Source: CAD feature listing. Evaluate the final solid. Frame: model axes, mm. Face numbers are marked on the shaded views. A direction names the side the tool comes from. Give positions to 0.01 mm unless a question says otherwise; leave off trailing zeros. Order: outer loops, then holes, each group sorted by start corner. A loop starts at its lowest first (then second) coordinate and runs counter-clockwise, first axis right, second up.
Autodesk Inventor part; units mm, degrees
ref_plane "Work Plane1" through (45, -30, 10) normal (0.7071, 0, -0.7071) x (0, 1, 0)
ref_plane "Work Plane2" through (0, 30, 0) normal (0, 1, 0) x (-1, 0, 0)
ref_plane "Work Plane3" through (0, -30, 0) normal (0, 1, 0) x (-1, 0, 0)
sketch "Sketch1" plane through (0, 0, 0) normal (0, 0, 1) x (1, 0, 0)
  line L0 (-363.8821, 101.7163) -> (-138.7473, 103.6763) construction
  line L1 (-138.7473, 103.6763) -> (-137.081, -87.7242) construction
  line L2 (-137.081, -87.7242) -> (-362.2158, -89.6841) construction
  line L3 (-362.2158, -89.6841) -> (-363.8821, 101.7163) construction
  line L4 (-45, 30) -> (45, 30)
  line L5 (45, 30) -> (45, -30)
  line L6 (-45, -30) -> (-45, 30)
  line L7 (-45, 30) -> (45, -30) construction
  line L8 (45, 30) -> (-45, -30) construction
  arc A0 (24, 0) -> (6, 0) centre (15, 0) ccw
  line L9 (15, 0) -> (6, 0) construction
  line L10 (15, 0) -> (24, 0) construction
  line L11 (6, 0) -> (6, -30)
  line L12 (24, 0) -> (24, -30)
  line L13 (45, -30) -> (24, -30)
  line L14 (6, -30) -> (-45, -30)
  point P0 (0, 0)
  dimension "d9" = 90
  dimension "d10" = 60
  dimension "d12" = 9
  dimension "d13" = 180
  dimension "d14" = 30
  dimension "d15" = 30
extrude "Extrusion1" add sketch "Sketch1" along normal blind 10
ref_plane "Work Plane1" through (45, -30, 10) normal (0.7071, 0, -0.7071) x (0, 1, 0)
sketch "Sketch2" plane through (45, -30, 10) normal (0.7071, 0, -0.7071) x (0, 1, 0)
  line L0 (60, 0) -> (60, -63.6396)
  line L1 (0, 0) -> (60, 0)
  circle A0 centre (30, 45.5) radius 7.5
  line L2 (60, 0) -> (36.9322, 55.8626)
  line L3 (0, 0) -> (23.0678, 55.8626)
  arc A1 (36.9322, 55.8626) -> (23.0678, 55.8626) centre (30, 53) ccw
  point P0 (30, -38.8909)
  dimension "d19" = 15
  dimension "d20" = 45.5
  dimension "d22" = 7.5
extrude "Extrusion2" add sketch "Sketch2" along normal blind 10
sketch "Sketch3" plane through (0, 0, 0) normal (0, 1, 0) x (-1, 0, 0)
  point P0 (0, 0)
sketch "Sketch4" plane through (0, 0, 0) normal (0, 0, 1) x (1, 0, 0)
  point P0 (0, 0)
sketch "Sketch5" plane through (0, 0, 0) normal (0, 1, 0) x (-1, 0, 0)
  point P0 (0, 0)
ref_plane "Work Plane2" through (0, 30, 0) normal (0, 1, 0) x (-1, 0, 0)
ref_plane "Work Plane3" through (0, -30, 0) normal (0, 1, 0) x (-1, 0, 0)
sketch "Sketch6" plane through (0, 30, 0) normal (0, 1, 0) x (-1, 0, 0)
  line L0 (-45, 0) -> (-45, 10)
  line L1 (-45, 10) -> (-52.0711, 2.9289)
  line L2 (-45, 0) -> (-52.0711, 2.9289)
  line L3 (-52.0711, 2.9289) -> (-45, 10)
  line L4 (-45, 10) -> (-45, 0)
  point P0 (0, 0)
sketch "Sketch7" plane through (0, -30, 0) normal (0, 1, 0) x (-1, 0, 0)
  point P0 (0, 0)
sketch "Sketch8" plane through (0, -30, 0) normal (0, 1, 0) x (-1, 0, 0)
  line L0 (-45, 10) -> (-52.0711, 2.9289)
  line L1 (-52.0711, 2.9289) -> (-45, 10)
  line L2 (-45, 0) -> (-45, 10)
  line L3 (-45, 10) -> (-45, 0)
  line L4 (-45, 0) -> (-52.0711, 2.9289)
  point P0 (0, 0)
loft "Loft1" add profiles "Sketch8", "Sketch6"
sketch "Sketch9" plane through (0, 0, 10) normal (0, 0, 1) x (1, 0, 0)
  line L0 (45, 30) -> (-45, 30)
  line L1 (-45, 30) -> (-105, 30)
  line L2 (-45, 30) -> (-45, -30)
  line L3 (-45, -30) -> (-105, -30)
  arc A0 (-45, -30) -> (-45, 30) centre (-45, 0) ccw
  arc A1 (-57, -9) -> (-57, 9) centre (-45, 0) ccw
  line L4 (-57, 9) -> (-105, 9)
  line L5 (-57, -9) -> (-105, -9)
  line L6 (-105, -30) -> (-105, -9)
  line L7 (-105, 9) -> (-105, 30)
  point P0 (0, 0)
  dimension "d31" = 60
  dimension "d32" = 60
  dimension "d33" = 15
  dimension "d34" = 18
  dimension "d35" = 21
extrude "Extrusion3" add sketch "Sketch9" along normal blind 17.5 and the other way blind 27.5 contours L2 A1 L4 L7 L1 | A0 L2 A1 | L3 L6 L5 A1 L2
sketch "Sketch10" plane through (-105, 9, 27.5) normal (-1, 0, 0) x (0, 0, 1)
  line L0 (-45, 0) -> (-45, 21)
  line L1 (0, 21) -> (0, 0)
  point P0 (-27.5, -9)
  point P1 (-45, 10.5)
  dimension "d40" = 45
sketch "Sketch11" plane through (-45, 30, 0) normal (0, 1, 0) x (1, 0, 0)
  circle A0 centre (-38.4851, -5) radius 12
  line L0 (0, -27.5) -> (-60, -27.5)
  point P0 (45, 0)
  dimension "d42" = 24
extrude "Extrusion4" cut sketch "Sketch11" against normal blind 9.5
sketch "Sketch12" plane through (-83.4851, 20.5, 5) normal (0, 1, 0) x (1, 0, 0)
  circle A0 centre (0, 0) radius 12
  circle A1 centre (0, 0) radius 6
  point P0 (83.4851, 5)
  dimension "d46" = 12
extrude "Extrusion5" cut sketch "Sketch12" against normal blind 12 contours A1
sketch "Sketch13" plane through (6, -30, 0) normal (0, -1, 0) x (1, 0, 0)
  circle A0 centre (-89.4851, 5) radius 12
  point P0 (-6, 0)
  dimension "d49" = 24
extrude "Extrusion6" cut sketch "Sketch13" against normal blind 9
sketch "Sketch14" plane through (-83.4851, -21, 5) normal (0, -1, 0) x (1, 0, 0)
  circle A0 centre (0, 0) radius 12
  circle A1 centre (0, 0) radius 6
  point P0 (83.4851, -5)
  dimension "d52" = 12
extrude "Extrusion7" cut sketch "Sketch14" against normal blind 12 contours A1
sketch "Sketch15" plane through (0, 0, 10) normal (0, 0, 1) x (1, 0, 0)
  arc A0 (-45, -15) -> (-45, 15) centre (-45, 0) ccw
  line L0 (-45, 15) -> (-45, -15)
  line L1 (-45, -15) -> (-45, 15)
  arc A1 (-45, -15) -> (-45, 15) centre (-45, 0) ccw
  point P0 (0, 0)
extrude "Extrusion8" cut sketch "Sketch15" against normal through all
properties part number "cad@40"
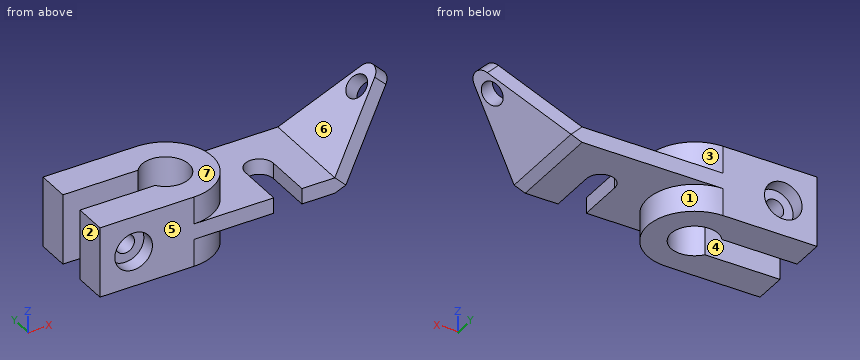
1) Pull-direction query (X, two-part tool) for the marked faces 1, 2 and 3; classes: +X half, -X half, draft (parallel to the pull), parting line (faces both ways), or undercut.
Checks:
face 1: +X half
face 2: -X half
face 3: undercut
2) First-contact query: pin 1 Ø6 at (x, z) = (47, 16.5) entering from +Y; pin 2 Ø13.5 at (x, z) = (-78.5, 5) entering from -Y; pin 3 Ø6 at (x, z) = (-33.5, -6) entering from +Y; pin 4 Ø1.5 at (y, z) = (-3, -7) entering from +X. Flat tips, straight axial feed; report the tip coordinate or a pass-through.
Checks:
pin 1: passes through
pin 2: stops at y = -21
pin 3: stops at y = 28.77
pin 4: stops at x = -15.08
3) Section query D-D on z = 23. Output: boundary loops of the cut face in (x, y).
Checks:
outline: (-105, -30) - (-45, -30) arc R30 ccw to (-45, 30) - (-105, 30) - (-105, 9) - (-57, 9) arc R15 cw (long way) to (-57, -9) - (-105, -9) - close; (58, -22.41) - (72.14, -18.28) - (72.14, 18.28) - (58, 22.41) - close
4) Reachability of the marked faces 4, 5, 6 and 7 from +Z, -Z, +X, -X, +Y, -Y: full face, straight path, thin tool, end or side. Return the list, or none.
Checks:
face 4: +Z, -Z, -X
face 5: +Z, -Z, +X, -X, -Y
face 6: +Z, +Y, -Y
face 7: +Z, -X, +Y, -Y
5) Ray query, L1, parallel to Y at x = -76, z = -6; L2, parallel to Z at x = 31, y = -23.5; L3, parallel to Y at x = -78, z = 11. Return the intervals inside material, ascending.
Checks:
L1: y = -30 to -9, 9 to 30
L2: z = 0 to 10
L3: y = -21 to -9, 9 to 20.5
6) Section query A-A on z = 5. State how many separate pieces and enclosed holes the cut face has, and give its area (3 significant figures).
Checks:
separate pieces: 3
enclosed holes: 0
area: 6,620 mm2
